Autodesk Inventor part; units mm, degrees
ref_plane "YZ Plane" through (0, 0, 0) normal (1, 0, 0) x (0, 1, 0)
ref_plane "XZ Plane" through (0, 0, 0) normal (0, 1, 0) x (-1, 0, 0)
ref_plane "XY Plane" through (0, 0, 0) normal (0, 0, 1) x (1, 0, 0)
sketch "Skizze1" plane through (0, 0, 0) normal (1, 0, 0) x (0, 1, 0)
  circle A0 centre (0, 0) radius 5
  circle A1 centre (0, 0) radius 10
  dimension "d0" = 10
  dimension "d3" = 5
extrude "Extrusion1" add sketch "Skizze1" along normal blind 30 contours A0
extrude "Extrusion2" add sketch "Skizze1" against normal blind 10 contours A0 | A1
fillet "Rundung1" radius 10 1 edges at (-10, -10, 0)
equation "\"d4\" = d3 + 0.5 * d0"
equation "\"d6\" = d3 + 0.5 * d0"
properties part number "FilmLamp-Clamp"
Design review of the part built by this model. Coordinates are the model's own, in mm. Give positions to 0.01 mm unless a question says otherwise; leave off trailing zeros. Loops run counter-clockwise (first coordinate to the right, second up) from the corner with the lowest first, then second, coordinate; pieces in that order, holes last. Notation, with made-up numbers: M 51.5,52.25 L 82.5,52.25 A24 cw 82.5,73.25 Z; hole C 20.25,70 d11. An arc over 180 degrees is marked long. Return JSON: item names as keys, results as strings. Group by question number.
Item 1: Insertion check: pin 1 Ø10 at (y, z) = (-7, -5) entering from -X; pin 2 Ø4 at (x, z) = (25.5, -6) entering from -Y; pin 3 Ø10 at (x, z) = (21.5, 6) entering from +Y; pin 4 Ø2 at (x, y) = (18.5, 6.5) entering from +Z. Each pin has a flat end and moves straight along its axis. Give the tip position at first contact, or say it passes through.
Item 2: For probe 1 along Y at (x, z) = (10, -0.5); probe 2 along X at (y, z) = (-6.25, 6.5), list the stretches that pass through material, from the lowest coordinate up.
Item 3: We need section A-A (x = 26.5). Give the boundary of the cut face in (y, z), and give its area (3 significant figures).
Item 4: Mouldability with a two-part tool opening along X and no side actions: class faces 1 (the flat face through (0, 2, 5)), 2 (the cylindrical face through (14.79, -1.08, 4.88)) as released by +X, released by -X, zero draft, split by the parting line, or undercut.
Output:
{
 "1": {"pin 1": "stops at x = -9.33", "pin 2": "stops at y = -3", "pin 3": "stops at y = 4.9", "pin 4": "passes through"},
 "2": {"probe 1": "y = -4.97 to 4.97", "probe 2": "x = -4.32 to 0"},
 "3": {"outline": "C 0,0 d10", "area": "78.5 mm^2"},
 "4": {"face 1": "released by +X", "face 2": "zero draft"}
}
